Input: part model. Units: mm. Frame: model coordinates. A direction names the side the tool comes from. Round coordinates to 2 decimals unless told otherwise and drop trailing zeros. Write each loop counter-clockwise with the first axis right and the second up, starting at its lowest first coordinate (ties: lowest second). Pieces come first, ordered by that corner, then holes. Notation, with made-up numbers: (15.25, 9) -> (31.25, 9) arc R38 ccw to (31.25, 48) -> close; hole circle Ø4 at (52.5, 42.25). An arc over 180 degrees is marked (long way). Write item = value, one per line.
Autodesk Fusion 360 part; units mm, degrees
sketch "スケッチ1" plane through (0, 0, 0) normal (0, 0, 1) x (1, 0, 0)
  line L0 (50, 30) -> (-50, 30)
  line L1 (-50, 30) -> (-50, -30)
  line L2 (-50, -30) -> (50, -30)
  line L3 (50, -30) -> (50, 30)
  line L4 (50, 30) -> (-50, -30) construction
  line L5 (-50, 30) -> (50, -30) construction
  line L6 (-40, 24) -> (-32, 24)
  line L7 (-32, 24) -> (-32, -24)
  line L8 (-32, -24) -> (-40, -24)
  line L9 (-40, -24) -> (-40, 24)
  line L10 (-50, 0) -> (50, 0) construction
  line L11 (0, -30) -> (0, 30) construction
  line L12 (-50, 24) -> (-44, 30)
  line L13 (-26, 30) -> (-19, 23)
  line L14 (-19, 23) -> (-13, 23)
  line L15 (-13, 23) -> (-9, 19)
  line L16 (-50, -24) -> (-44, -30)
  line L17 (-26, -30) -> (-19, -23)
  line L18 (-19, -23) -> (-13, -23)
  line L19 (-13, -23) -> (-9, -19)
  line L20 (50, 24) -> (44, 30)
  line L21 (26, 30) -> (19, 23)
  line L22 (19, 23) -> (13, 23)
  line L23 (13, 23) -> (9, 19)
  line L24 (13, -23) -> (9, -19)
  line L25 (19, -23) -> (13, -23)
  line L26 (26, -30) -> (19, -23)
  line L27 (50, -24) -> (44, -30)
  line L28 (-9, 19) -> (9, 19)
  line L29 (-10, 25) -> (10, 25)
  line L30 (-10, 25) -> (-11, 21)
  line L31 (10, 25) -> (11, 21)
  line L32 (-10, -25) -> (-11, -21)
  line L33 (-10, -25) -> (10, -25)
  line L34 (10, -25) -> (11, -21)
  line L35 (-9, -19) -> (9, -19)
  line L36 (40, 24) -> (32, 24)
  line L37 (40, -24) -> (40, 24)
  line L38 (32, 24) -> (32, -24)
  line L39 (32, -24) -> (40, -24)
  dimension "d1" = 100
  dimension "d2" = 60
  dimension "d3" = 8
  dimension "d4" = 48
  dimension "d5" = 10
  dimension "d6" = 6
  dimension "d7" = 6
  dimension "d8" = 18
  dimension "d9" = 7
  dimension "d10" = 7
  dimension "d11" = 6
  dimension "d12" = 4
  dimension "d13" = 4
  dimension "d14" = 6
  dimension "d15" = 20
extrude "押し出し1" add sketch "スケッチ1" along normal blind 4 contours L0 L1 L2 L3 L12 L13 L14 L15 L16 L17 L18 L19 L20 L21 L22 L23 L24 L25 L26 L27 L28 L35
extrude "押し出し2" add sketch "スケッチ1" along normal blind 3 contours L15 L23 L28 L29 L30 L31 | L19 L24 L32 L33 L34 L35
fillet "フィレット1" radius 1 16 edges at (-11, -21, 1.5) (-9, -19, 3.5) (11, -21, 1.5) (9, -19, 3.5) (11, 21, 1.5) (9, 19, 3.5) (-9, 19, 3.5) (-11, 21, 1.5) (32, -24, 2) (40, -24, 2) (-40, 24, 2) (-32, 24, 2) (40, 24, 2) (32, 24, 2) (-32, -24, 2) (-40, -24, 2)
fillet "フィレット2" radius 1 4 edges at (-19, -23, 2) (19, -23, 2) (19, 23, 2) (-19, 23, 2)
fillet "フィレット3" radius 1 12 edges at (-26, 30, 2) (-44, 30, 2) (-50, 24, 2) (-50, -24, 2) (-44, -30, 2) (-26, -30, 2) (26, -30, 2) (44, -30, 2) (50, -24, 2) (26, 30, 2) (44, 30, 2) (50, 24, 2)
fillet "フィレット4" radius 1 4 edges at (10, -25, 1.5) (-10, -25, 1.5) (-10, 25, 1.5) (10, 25, 1.5)
equation "d7 = d6"
1) First-contact query: P1, Ø1.2, axis at x = 17, z = 1, coming from the -Y side; P2, Ø0.8, axis at x = -3, z = 3.5, coming from the -Y side; P3, Ø1.8, axis at x = -5.5, y = -22.5, coming from the +Z side. Flat tips, straight axial feed; report the tip coordinate or a pass-through.
Solutions:
P1 = -23
P2 = -19
P3 = 3
2) Cut plane B-B (x = -20.5). Return the cut outline in (y, z), and give its area (3 significant figures).
Solutions:
outline = (-24.5, 0) -> (24.5, 0) -> (24.5, 4) -> (-24.5, 4) -> close
area = 196 mm^2
3) Cut plane C-C (z = 2.1). Count the separate pieces of the cut face and the enclosed holes in it, and give its area (3 significant figures).
Solutions:
separate_pieces = 1
enclosed_holes = 2
area = 4,610 mm^2
4) Cut plane A-A (y = 9). Return the cut outline in (x, z).
Solutions:
outline = (-50, 0) -> (-40, 0) -> (-40, 4) -> (-50, 4) -> close; (-32, 0) -> (32, 0) -> (32, 4) -> (-32, 4) -> close; (40, 0) -> (50, 0) -> (50, 4) -> (40, 4) -> close
5) Draft query along Y for faces 1 (the face through (-40, 0, 2)), 2 (the face through (-1, 0, 0)), 3 (the face through (36, 24, 2)), 4 (the face through (-47, -27, 2)). Return one class per face: +Y half, -Y half, draft (parallel to the pull), parting line (faces both ways), or undercut.
Solutions:
face_1 = undercut
face_2 = draft
face_3 = undercut
face_4 = -Y half
6) Line query: L1, parallel to X at y = -14, z = 0.8; L2, parallel to Y at x = 37, z = 1.8; L3, parallel to X at y = -20, z = 3.5. Output: solid intervals per line, ascending. Write a range as from..to.
Solutions:
L1 = -50..-40, -32..32, 40..50
L2 = -30..-24, 24..30
L3 = -50..-40, -32..-10, 10..32, 40..50
7) Access query for faces 5 (the face through (-32, 0, 2)), 6 (the face through (0, 22, 3)), 7 (the face through (-23, -27, 2)). Directions: +Z, -Z, +X, -X, +Y, -Y. A direction counts if a zero-diameter tool reaches every point of the face in a straight line with its end or side. Return the directions, or none.
Solutions:
face_5 = +Z, -Z
face_6 = +Z, +Y
face_7 = +Z, -Z, -Y
